```python
from build123d import *

# Parameters (mm, degrees)
SKETCH_1_W          = 20
SKETCH_1_H          = 53
EXTRUDE_1_DEPTH     = 3
SKETCH_2_W          = 70
SKETCH_2_H          = 20
EXTRUDE_2_DEPTH     = 3
SKETCH_3_R          = 1.6
CUT_EXTRUDE_1_DEPTH = 70.591666168
FILLET_1_R          = 10
FILLET_2_R          = 5


with BuildPart() as part:
    # 草图1 → 凸台-拉伸1 (new body)
    with BuildSketch(Plane.XY):
        with Locations((10, 26.5)):
            Rectangle(SKETCH_1_W, SKETCH_1_H)
    extrude(amount=EXTRUDE_1_DEPTH)

    # 草图2 → 凸台-拉伸2 (add)
    with BuildSketch(Plane.XY.offset(3)):
        with Locations((10, 10)):
            Rectangle(SKETCH_2_W, SKETCH_2_H)
    extrude(amount=-EXTRUDE_2_DEPTH)

    # 草图3 → 切除-拉伸1 (cut, through all)
    with BuildSketch(Plane.XY.offset(3)):
        with Locations((10, 48)):
            Circle(SKETCH_3_R)
        with Locations((10, 30)):
            Circle(SKETCH_3_R)
        with Locations((10, 10)):
            Circle(SKETCH_3_R)
        with Locations((-15, 10)):
            Circle(SKETCH_3_R)
        with Locations((35, 10)):
            Circle(SKETCH_3_R)
    extrude(amount=-CUT_EXTRUDE_1_DEPTH, mode=Mode.SUBTRACT)

    # 圆角1
    fillet_1_edges = [part.edges().sort_by_distance(p)[0] for p in [
        (0, 20, 1.5),
        (20, 20, 1.5),
    ]]
    fillet(fillet_1_edges, radius=FILLET_1_R)

    # 圆角2
    fillet_2_edges = [part.edges().sort_by_distance(p)[0] for p in [
        (-25, 20, 1.5),
        (45, 0, 1.5),
        (-25, 0, 1.5),
        (45, 20, 1.5),
        (0, 53, 1.5),
        (20, 53, 1.5),
    ]]
    fillet(fillet_2_edges, radius=FILLET_2_R)


solid = part.part
```
Geometry check sheet. Reference: the model listing, model coordinates, mm. A direction names the side the tool comes from. Coordinates: 2 decimals unless noted, no trailing zeros. Write each loop counter-clockwise with the first axis right and the second up, starting at its lowest first coordinate (ties: lowest second). Pieces come first, ordered by that corner, then holes. Notation, with made-up numbers: M 59,63.5 L 84,63.5 A31 ccw 84,94.5 Z; hole C -14,42.5 d10. An arc over 180 degrees is marked long. Answer as a JSON object with one key per item and string values.
1. Section check D-D, the plane x = 10. Enter the section's corners in (y, z).
Answers below:
{"outline": "M 0,0 L 8.4,0 L 8.4,3 L 0,3 Z; M 11.6,0 L 28.4,0 L 28.4,3 L 11.6,3 Z; M 31.6,0 L 46.4,0 L 46.4,3 L 31.6,3 Z; M 49.6,0 L 53,0 L 53,3 L 49.6,3 Z"}
2. Section check C-C, the plane z = 2.1. Enter the section's corners in (x, y).
Answers below:
{"outline": "M -25,5 A5 ccw -20,0 L 40,0 A5 ccw 45,5 L 45,15 A5 ccw 40,20 L 30,20 A10 cw 20,30 L 20,48 A5 ccw 15,53 L 5,53 A5 ccw 0,48 L 0,30 A10 cw -10,20 L -20,20 A5 ccw -25,15 Z; hole C -15,10 d3.2; hole C 10,10 d3.2; hole C 10,30 d3.2; hole C 10,48 d3.2; hole C 35,10 d3.2"}
3. Go/stop test with flat-tipped pins: pin 1 Ø0.9 at (y, z) = (35, 1) entering from -X; pin 2 Ø0.9 at (y, z) = (37, 1.5) entering from +X; pin 3 Ø1.9 at (x, y) = (-15, 10) entering from -Z; pin 4 Ø1.5 at (x, z) = (34.5, 1.5) entering from +Y. Record where each tip stops, or that it passes through.
Answers below:
{"pin 1": "stops at x = 0", "pin 2": "stops at x = 20", "pin 3": "passes through", "pin 4": "stops at y = 20"}
4. Scan lines: L1, parallel to Y at x = 10, z = 2.25; L2, parallel to Y at x = -13, z = 2.55; L3, parallel to Y at x = 35, z = 1.5. Record each from-to range of solid material in increasing order.
Answers below:
{"L1": "y = 0 to 8.4, 11.6 to 28.4, 31.6 to 46.4, 49.6 to 53", "L2": "y = 0 to 20", "L3": "y = 0 to 8.4, 11.6 to 20"}
5. Section check B-B, the plane x = -15. Enter the section's corners in (y, z), plus the area to 3 significant figures.
Answers below:
{"outline": "M 0,0 L 8.4,0 L 8.4,3 L 0,3 Z; M 11.6,0 L 20,0 L 20,3 L 11.6,3 Z", "area": "50.4 mm²"}
6. Section check A-A, the plane y = 10. Enter the section's corners in (x, z), plus the area to 3 significant figures.
Answers below:
{"outline": "M -25,0 L -16.6,0 L -16.6,3 L -25,3 Z; M -13.4,0 L 8.4,0 L 8.4,3 L -13.4,3 Z; M 11.6,0 L 33.4,0 L 33.4,3 L 11.6,3 Z; M 36.6,0 L 45,0 L 45,3 L 36.6,3 Z", "area": "181 mm²"}
7. Tool access check on faces 1 (the flat face through (20, 39, 1)), 2 (the flat face through (10, 21, 0)), 3 (the flat face through (0, 39, 1)). Record the directions out of +Z, -Z, +X, -X, +Y, -Y that give a thin tool (end or side, any length) a straight path to the whole face; none if there is none.
Answers below:
{"face 1": "+Z, -Z, +X, +Y", "face 2": "-Z, +X, -X, +Y, -Y", "face 3": "+Z, -Z, -X, +Y"}
